```python
from build123d import *

# Parameters (mm, degrees)
ESBO_O1_W                = 5
ESBO_O1_H                = 6
RESSALTO_EXTRUS_O1_DEPTH = 1
ESBO_O2_W                = 5
ESBO_O2_H                = 1
RESSALTO_EXTRUS_O2_DEPTH = 5
CORTE_EXTRUS_O1_REACH    = 8
CORTE_EXTRUS_O2_REACH    = 3
ESBO_O4_R                = 1
CORTE_EXTRUS_O3_REACH    = 3
ESBO_O5_R                = 1


with BuildPart() as part:
    # Esboço1 → Ressalto-extrusão1 (new body)
    with BuildSketch(Plane.XY):
        Rectangle(ESBO_O1_W, ESBO_O1_H)
    extrude(amount=-RESSALTO_EXTRUS_O1_DEPTH)

    # Esboço2 → Ressalto-extrusão2 (add)
    with BuildSketch(Plane(origin=(0, 0, -1), x_dir=(-1, 0, 0), z_dir=(0, 0, -1))):
        with Locations((0, -2.5)):
            Rectangle(ESBO_O2_W, ESBO_O2_H)
    extrude(amount=RESSALTO_EXTRUS_O2_DEPTH)

    # Esboço3 → Corte-extrusão1 (cut, up to next)
    with BuildSketch(Plane.XY, mode=Mode.PRIVATE) as corte_extrus_o1_sk1:
        with BuildLine():
            ThreePointArc((3.35e-07, -3), (-1.250125983, -2.991119921), (-2.5, -2.964481468))
            Line((-2.5, -2.964481468), (-2.5, -3))
            Line((-2.5, -3), (3.35e-07, -3))
        make_face()
    corte_extrus_o1_tool1 = extrude(corte_extrus_o1_sk1.sketch, amount=-CORTE_EXTRUS_O1_REACH, mode=Mode.PRIVATE) & part.part
    add(corte_extrus_o1_tool1.solids().sort_by_distance((-1.875025, -2.989345, 0))[0], mode=Mode.SUBTRACT)
    # Esboço3 → Corte-extrusão1 (cut, up to next)
    with BuildSketch(Plane.XY, mode=Mode.PRIVATE) as corte_extrus_o1_sk2:
        with BuildLine():
            Line((2.5, -3), (2.5, -2.964481468))
            ThreePointArc((2.5, -2.964481468), (1.250126318, -2.991119917), (3.35e-07, -3))
            Line((3.35e-07, -3), (2.5, -3))
        make_face()
    corte_extrus_o1_tool2 = extrude(corte_extrus_o1_sk2.sketch, amount=-CORTE_EXTRUS_O1_REACH, mode=Mode.PRIVATE) & part.part
    add(corte_extrus_o1_tool2.solids().sort_by_distance((1.875025, -2.989345, 0))[0], mode=Mode.SUBTRACT)

    # Esboço4 → Corte-extrusão2 (cut, up to next)
    with BuildSketch(Plane(origin=(0, -2, 0), x_dir=(1, 0, 0), z_dir=(0, 1, 0)), mode=Mode.PRIVATE) as corte_extrus_o2_sk1:
        with Locations((0, 3.5)):
            Circle(ESBO_O4_R)
    corte_extrus_o2_tool1 = extrude(corte_extrus_o2_sk1.sketch, amount=-CORTE_EXTRUS_O2_REACH, mode=Mode.PRIVATE) & part.part
    add(corte_extrus_o2_tool1.solids().sort_by_distance((0, -2, -3.5))[0], mode=Mode.SUBTRACT)

    # Esboço5 → Corte-extrusão3 (cut, up to next)
    with BuildSketch(Plane(origin=(0, 0, -1), x_dir=(-1, 0, 0), z_dir=(0, 0, -1)), mode=Mode.PRIVATE) as corte_extrus_o3_sk1:
        with Locations((0, 0.5)):
            Circle(ESBO_O5_R)
    corte_extrus_o3_tool1 = extrude(corte_extrus_o3_sk1.sketch, amount=-CORTE_EXTRUS_O3_REACH, mode=Mode.PRIVATE) & part.part
    add(corte_extrus_o3_tool1.solids().sort_by_distance((0, 0.5, -1))[0], mode=Mode.SUBTRACT)


solid = part.part
```
Verification items for the finished model (mm, model axes). A direction names the side the tool comes from. Give positions to 0.01 mm unless a question says otherwise; leave off trailing zeros. Write each loop counter-clockwise with the first axis right and the second up, starting at its lowest first coordinate (ties: lowest second). Pieces come first, ordered by that corner, then holes. Notation, with made-up numbers: (58, -6) - (88, -6) arc R8 cw to (88, 6) - close; hole circle Ø10 at (-0.75, 63.5). An arc over 180 degrees is marked (long way). Put each result on its own line as item: value.
Q1. Scan lines: probe 1 along X at (y, z) = (-2.7, -3.5); probe 2 along Z at (x, y) = (0, -2.5); probe 3 along Z at (x, y) = (1.55, 0). Record each from-to range of solid material in increasing order. Write a range as from..to.
Result:
probe 1: -2.5..-1, 1..2.5
probe 2: -6..-4.5, -2.5..0
probe 3: -1..0
Q2. Section check B-B on z = -0.5. Record the cut outline in (x, y), and give its area (3 significant figures).
Result:
outline: (-2.5, -2.96) arc R88 ccw to (0, -3) arc R88 ccw to (2.5, -2.96) - (2.5, 3) - (-2.5, 3) - close; hole circle Ø2 at (0, 0.5)
area: 26.8 mm2
Q3. Mould release check, pull along X, two halves, no side actions. Record for faces 3 (the face through (0.217, -0.476, -0.507)), 4 (the face through (0, -1, 0)): released by +X, released by -X, zero draft, split by the parting line, or undercut.
Result:
face 3: undercut
face 4: zero draft
Q4. Section check A-A on y = 0.5. Record the cut outline in (x, z), and give its area (3 significant figures).
Result:
outline: (-2.5, -1) - (-1, -1) - (-1, 0) - (-2.5, 0) - close; (1, -1) - (2.5, -1) - (2.5, 0) - (1, 0) - close
area: 3.00 mm2
Q5. Set-up check for faces 1 (the face through (0, 2, -1)), 2 (the face through (-0.13, -2.49, -4.49)): record each of +Z, -Z, +X, -X, +Y, -Y from which the full face is reachable in a straight line by a thin tool's end or side.
Result:
face 1: -Z, +X, -X, +Y
face 2: +Y, -Y
Q6. Section check C-C on x = -0.65. Record the cut outline in (y, z), and give its area (3 significant figures).
Result:
outline: (-3, -6) - (-2, -6) - (-2, -4.26) - (-3, -4.26) - close; (-3, -2.74) - (-2, -2.74) - (-2, -1) - (-0.26, -1) - (-0.26, 0) - (-3, 0) - close; (1.26, -1) - (3, -1) - (3, 0) - (1.26, 0) - close
area: 7.95 mm2
Q7. Section check D-D on z = -3.5. Record the cut outline in (x, y).
Result:
outline: (-2.5, -2.96) arc R88 ccw to (-1, -2.99) - (-1, -2) - (-2.5, -2) - close; (1, -2.99) arc R88 ccw to (2.5, -2.96) - (2.5, -2) - (1, -2) - close
Q8. Depth check by flat-ended pin: P1, Ø2.5, axis at x = -0.5, z = -3, coming from the +Y side; P2, Ø1, axis at x = 1.5, z = -4.5, coming from the -Y side. Enter the tip coordinate at first touch or a pass-through.
Result:
P1: y = -2
P2: y = -2.99
